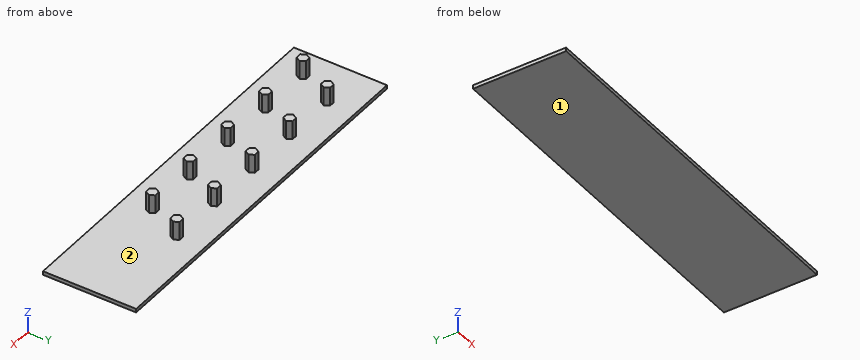
```python
from build123d import *

# Parameters (mm, degrees)
F0_W     = 508
F0_H     = 127
F1_DEPTH = 5.08
F3_DEPTH = 25.4


with BuildPart() as f1:
    # F0 (on Top) → F1 (new body)
    with BuildSketch(Plane.XY):
        with Locations((254, 63.5)):
            Rectangle(F0_W, F0_H)
    extrude(amount=F1_DEPTH)

    # F2 (on face) → F3 (join)
    with BuildSketch(Plane.XY.offset(5.08)):
        Polygon((45.356168, 38.303634), (41.551732, 44.485843), (34.295564, 44.282209), (30.843832, 37.896366), (34.648268, 31.714157), (41.904436, 31.917791), align=None)
        Polygon((67.903701, 82.609158), (71.54074, 88.891306), (67.91876, 95.182149), (60.65974, 95.190842), (57.022701, 88.908694), (60.644682, 82.617851), align=None)
        Polygon((144.11876, 95.182149), (136.85974, 95.190842), (133.222701, 88.908694), (136.844682, 82.617851), (144.103701, 82.609158), (147.74074, 88.891306), align=None)
        Polygon((110.848268, 31.714157), (118.104436, 31.917791), (121.556168, 38.303634), (117.751732, 44.485843), (110.495564, 44.282209), (107.043832, 37.896366), align=None)
        Polygon((220.31876, 95.182149), (213.05974, 95.190842), (209.422701, 88.908694), (213.044682, 82.617851), (220.303701, 82.609158), (223.94074, 88.891306), align=None)
        Polygon((187.048268, 31.714157), (194.304436, 31.917791), (197.756168, 38.303634), (193.951732, 44.485843), (186.695564, 44.282209), (183.243832, 37.896366), align=None)
        Polygon((296.51876, 95.182149), (289.25974, 95.190842), (285.622701, 88.908694), (289.244682, 82.617851), (296.503701, 82.609158), (300.14074, 88.891306), align=None)
        Polygon((263.248268, 31.714157), (270.504436, 31.917791), (273.956168, 38.303634), (270.151732, 44.485843), (262.895564, 44.282209), (259.443832, 37.896366), align=None)
        Polygon((372.71876, 95.182149), (365.45974, 95.190842), (361.822701, 88.908694), (365.444682, 82.617851), (372.703701, 82.609158), (376.34074, 88.891306), align=None)
        Polygon((339.448268, 31.714157), (346.704436, 31.917791), (350.156168, 38.303634), (346.351732, 44.485843), (339.095564, 44.282209), (335.643832, 37.896366), align=None)
    extrude(amount=F3_DEPTH)


solid = f1.part
```
Check sheet for the modelled part. Datum: model origin and axes. Units: mm. Face numbers are marked on the shaded views. Round coordinates to 2 decimals unless told otherwise and drop trailing zeros. Order: outer loops, then holes, each group sorted by start corner. A loop starts at its lowest first (then second) coordinate and runs counter-clockwise, first axis right, second up.
1) Section check C-C (x = 427.5). Record the boundary of the cut face in (y, z).
2) Go/stop test with flat-tipped pins: pin 1 Ø5 at (x, z) = (74, 15.5) entering from +Y; pin 2 Ø2 at (x, y) = (196.5, 91.5) entering from +Z; pin 3 Ø8 at (x, z) = (69.5, 12.5) entering from -Y. Record where each tip stops, or that it passes through.
3) Mould release check, pull along Z, two halves, no side actions. Record for the marked faces 1 and 2: +Z half, -Z half, draft (parallel to the pull), parting line (faces both ways), or undercut.
4) Scan lines: line 1 (X direction, y = 36, z = 27); line 2 (X direction, y = 32.5, z = 14); line 3 (Z direction, x = 296.5, y = 11.5). Record each from-to range of solid material in increasing order.
5) Section check B-B (y = 26). Record the boundary of the cut face in (x, z).
6) Section check A-A (z = 12.5). Give the number of separate pieces and of enclosed holes in the cut face, and give its area (3 significant figures).
Result:
1. outline: (0, 0) - (127, 0) - (127, 5.08) - (0, 5.08) - close
2. pin 1: stops at y = 88.96
2. pin 2: stops at z = 5.08
2. pin 3: stops at y = 82.61
3. face 1: -Z half
3. face 2: +Z half
4. line 1: x = 32.01 to 44.11, 108.21 to 120.31, 184.41 to 196.51, 260.61 to 272.71, 336.81 to 348.91
4. line 2: x = 34.16 to 42.22, 110.36 to 118.42, 186.56 to 194.62, 262.76 to 270.82, 338.96 to 347.02
4. line 3: z = 0 to 5.08
5. outline: (0, 0) - (508, 0) - (508, 5.08) - (0, 5.08) - close
6. separate pieces: 10
6. enclosed holes: 0
6. area: 1,370 mm2
